Design review of the part built by this model. Coordinates are the model's own, in mm. Face numbers are marked on the shaded views. Coordinates: 2 decimals unless noted, no trailing zeros. Loops run counter-clockwise (first coordinate to the right, second up) from the corner with the lowest first, then second, coordinate; pieces in that order, holes last. Notation, with made-up numbers: (4.25, 21) -> (50.25, 21) arc R21 cw to (50.25, 41) -> close; hole circle Ø4 at (-11, 26.25). An arc over 180 degrees is marked (long way). One line per item, written item: value. Start each with the question number.
1. Draft analysis for pull direction Y (two halves, no side actions). For the marked faces 1, 2, 3 and 4, state which applies: pulls with the +Y half, pulls with the -Y half, needs draft (parallel to the pull), parting line crosses it, or undercut.
2. Add section D-D on y = 16. Give the number of separate pieces and of enclosed holes in the cut face, plus the area to 3 significant figures.
3. Add section A-A on x = 0. Write out the cut boundary in (y, z), plus the area to 3 significant figures.
4. For probe 1 along X at (y, z) = (-25, 11); probe 2 along Z at (x, y) = (46, 27.5); probe 3 along Y at (x, z) = (-58, 6.25), list the stretches that pass through material, from the lowest coordinate up.
5. Insertion check: pin 1 (4 mm diameter, centred on x = 33.5, z = 11.5, fed in from +Y); pin 2 (4 mm diameter, centred on y = -41, z = 4.5, fed in from -X); pin 3 (4 mm diameter, centred on x = -12.5, z = 6.5, fed in from +Y); pin 4 (1 mm diameter, centred on x = -29, y = 48.5, fed in from -Z). Each pin has a flat end and moves straight along its axis. Give the tip position at first contact, or say it passes through.
6. Add section C-C on z = 11. Write out the cut boundary in (x, y).
7. Add section B-B on y = -11.5. Write out the cut boundary in (x, z).
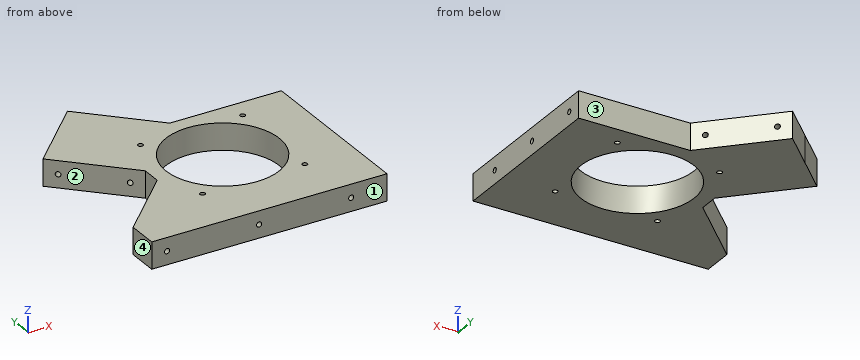
```python
from build123d import *

# Parameters (mm, degrees)
SKETCH1_R           = 27.7
SKETCH1_R_2         = 1.25
BOSS_EXTRUDE1_DEPTH = 13
CUT_EXTRUDE1_REACH  = 107.038
SKETCH2_R           = 1.25
SKETCH3_R           = 1.25
CUT_EXTRUDE2_DEPTH  = 15
SKETCH4_R           = 1.25
CUT_EXTRUDE3_DEPTH  = 15


with BuildPart() as part:
    # Sketch1 → Boss-Extrude1 (new body)
    with BuildSketch(Plane.XY):
        Polygon((50, 35), (50, -50), (-65, -50), (-65, -35), (-35, -5), (-35, 4.594408409), (-66.114484041, 35.70889245), (-50.911688245, 50.911688245), (-35.70889245, 66.114484041), (-4.594408409, 35), align=None)
        with Locations(Location((0, 0, 0), (0, 0, 180))):
            Circle(SKETCH1_R, mode=Mode.SUBTRACT)
        with Locations(Location((-25, 25, 0), (0, 0, 180))):
            Circle(SKETCH1_R_2, mode=Mode.SUBTRACT)
        with Locations(Location((25, 25, 0), (0, 0, 180))):
            Circle(SKETCH1_R_2, mode=Mode.SUBTRACT)
        with Locations(Location((25, -25, 0), (0, 0, 180))):
            Circle(SKETCH1_R_2, mode=Mode.SUBTRACT)
        with Locations(Location((-25, -25, 0), (0, 0, 180))):
            Circle(SKETCH1_R_2, mode=Mode.SUBTRACT)
    extrude(amount=BOSS_EXTRUDE1_DEPTH)

    # Sketch2 → Cut-Extrude1 (cut, up to next)
    with BuildSketch(Plane(origin=(-15.202795796, -15.202795796, 0), x_dir=(0, 0, 1), z_dir=(-0.7071067811865472, -0.7071067811865478, 0)), mode=Mode.PRIVATE) as cut_extrude1_sk1:
        with Locations(Location((6.5, 65.5, 0), (0, 0, 270))):
            Circle(SKETCH2_R)
    cut_extrude1_tool1 = extrude(cut_extrude1_sk1.sketch, amount=-CUT_EXTRUDE1_REACH, mode=Mode.PRIVATE) & part.part
    # Sketch2 → Cut-Extrude1 (cut, up to next)
    with BuildSketch(Plane(origin=(-15.202795796, -15.202795796, 0), x_dir=(0, 0, 1), z_dir=(-0.7071067811865472, -0.7071067811865478, 0)), mode=Mode.PRIVATE) as cut_extrude1_sk2:
        with Locations(Location((6.5, 34.5, 0), (0, 0, 270))):
            Circle(SKETCH2_R)
    cut_extrude1_tool2 = extrude(cut_extrude1_sk2.sketch, amount=-CUT_EXTRUDE1_REACH, mode=Mode.PRIVATE) & part.part
    add(cut_extrude1_tool1.solids().sort_by_distance((-61.51829, 31.112698, 6.5))[0], mode=Mode.SUBTRACT)
    add(cut_extrude1_tool2.solids().sort_by_distance((-39.59798, 9.192388, 6.5))[0], mode=Mode.SUBTRACT)

    # Sketch3 → Cut-Extrude2 (cut)
    with BuildSketch(Plane.XZ.offset(50)):
        with Locations((-57.5, 6.5)):
            Circle(SKETCH3_R)
        with Locations((32.5, 6.5)):
            Circle(SKETCH3_R)
        with Locations((-12.5, 6.5)):
            Circle(SKETCH3_R)
    extrude(amount=-CUT_EXTRUDE2_DEPTH, mode=Mode.SUBTRACT)

    # Sketch4 → Cut-Extrude3 (cut)
    with BuildSketch(Plane(origin=(50, 0, 0), x_dir=(0, 0, -1), z_dir=(1, 0, 0))):
        with Locations(Location((-6.5, -32.5, 0), (0, 0, 90))):
            Circle(SKETCH4_R)
        with Locations(Location((-6.5, 27.5, 0), (0, 0, 90))):
            Circle(SKETCH4_R)
        with Locations(Location((-6.5, -2.5, 0), (0, 0, 90))):
            Circle(SKETCH4_R)
    extrude(amount=-CUT_EXTRUDE3_DEPTH, mode=Mode.SUBTRACT)


solid = part.part
```
Worked answers:
1. face 1: pulls with the -Y half
1. face 2: undercut
1. face 3: pulls with the +Y half
1. face 4: needs draft
2. separate pieces: 2
2. enclosed holes: 1
2. area: 658 mm²
3. outline: (-50, 0) -> (-27.7, 0) -> (-27.7, 13) -> (-50, 13) -> close; (27.7, 0) -> (35, 0) -> (35, 13) -> (27.7, 13) -> close
3. area: 385 mm²
4. probe 1: x = -55 to -26.25, -23.75 to -11.93, 11.93 to 23.75, 26.25 to 50
4. probe 2: z = 0 to 5.25, 7.75 to 13
4. probe 3: y = -35 to -28, 27.59 to 32.9, 36.36 to 43.82
5. pin 1: stops at y = 35
5. pin 2: stops at x = -65
5. pin 3: stops at y = 44.91
5. pin 4: stops at z = 0
6. outline: (-66.11, 35.71) -> (-35, 4.59) -> (-35, -5) -> (-65, -35) -> (-65, -50) -> (50, -50) -> (50, 35) -> (-4.59, 35) -> (-35.71, 66.11) -> close; hole circle Ø55.4 at (0, 0); hole circle Ø2.5 at (-25, -25); hole circle Ø2.5 at (-25, 25); hole circle Ø2.5 at (25, -25); hole circle Ø2.5 at (25, 25)
7. outline: (-41.5, 0) -> (-25.2, 0) -> (-25.2, 13) -> (-41.5, 13) -> close; (25.2, 0) -> (50, 0) -> (50, 13) -> (25.2, 13) -> close
